Input: part model. Units: mm. Frame: model coordinates. A direction names the side the tool comes from. Give positions to 0.01 mm unless a question says otherwise; leave off trailing zeros. Loops run counter-clockwise (first coordinate to the right, second up) from the corner with the lowest first, then second, coordinate; pieces in that order, holes last. Notation, with made-up numbers: (-10, -38) -> (4, -38) arc R7 ccw to (4, -34) -> close; hole circle Ø3 at (18, -25). An arc over 180 degrees is marked (long way). Answer in a Markdown table with one row per item. Add a question column.
```python
from build123d import *

# Parameters (mm, degrees)
F0_R     = 0.3937
F1_DEPTH = 0.1778
F2_DEPTH = 1.143
F3_DEPTH = 1.524
F4_SCALE = 7.5


with BuildPart() as f1:
    # F0 (on Front) → F1 (new body, symmetric)
    with BuildSketch(Plane.XZ):
        with BuildLine():
            ThreePointArc((0, 8.2042), (-0.4130917816, 8.0330917816), (-0.5842, 7.62))
            Line((-0.5842, 7.62), (-0.5842, 0))
            ThreePointArc((-0.5842, 0), (-0.4130917816, -0.4130917816), (0, -0.5842))
            ThreePointArc((0, -0.5842), (0.4130917816, -0.4130917816), (0.5842, 0))
            Line((0.5842, 0), (0.5842, 7.62))
            ThreePointArc((0.5842, 7.62), (0.4130917816, 8.0330917816), (0, 8.2042))
        make_face()
        Circle(F0_R, mode=Mode.SUBTRACT)
        with BuildLine():
            ThreePointArc((-0.3937, 7.62), (0, 8.0137), (0.3937, 7.62))
            ThreePointArc((0.3937, 7.62), (0, 7.2263), (-0.3937, 7.62))
        make_face(mode=Mode.SUBTRACT)
    extrude(amount=F1_DEPTH, both=True)

    # F0 (on Front) → F2 (join, symmetric)
    with BuildSketch(Plane.XZ):
        Circle(F0_R)
    extrude(amount=F2_DEPTH, both=True)

    # F0 (on Front) → F3 (join)
    with BuildSketch(Plane.XZ):
        with BuildLine():
            ThreePointArc((-0.3937, 7.62), (0, 7.2263), (0.3937, 7.62))
            ThreePointArc((0.3937, 7.62), (0, 8.0137), (-0.3937, 7.62))
        make_face()
    extrude(amount=-F3_DEPTH)


with BuildPart() as f1_1:
    # F4: moved
    add(f1.part.scale(F4_SCALE))


solid = f1_1.part
```
1) Section B-B on x = -2.25. Output: boundary loops of the cut face in (y, z).
2) Section A-A on y = -0.75. Output: boundary loops of the cut face in (x, z).
3) Pull-direction query (Z, two-part tool) for faces 5 (the face through (-2.34, -5, -1.8)), 6 (the face through (0, 11.43, 57)), 7 (the face through (0, 0, 57)); classes: +Z half, -Z half, draft (parallel to the pull), parting line (faces both ways), or undercut.
4) Section C-C on y = 2. Output: boundary loops of the cut face in (x, z), and give its area (3 significant figures).
5) Section D-D on z = 29.5. Output: boundary loops of the cut face in (x, y), and give its area (3 significant figures).
6) Pin query (flat end, axial travel): pin 1 (2 mm diameter, centred on x = -1, y = 2.5, fed in from +Z); pin 2 (1 mm diameter, centred on x = -1.5, y = -1.5, fed in from +Z); pin 3 (2 mm diameter, centred on x = 3, z = 26.5, fed in from +Y). Return the tip coordinate at first contact, or that it passes through.
7) Reachability of faces 1 (the face through (-0.64, -0.657, 60.033)), 2 (the face through (-2.34, 4.9, -1.8)), 3 (the face through (0, 8.572, 0)), 4 (the face through (0, -8.572, 0)) from +Z, -Z, +X, -X, +Y, -Y: full face, straight path, thin tool, end or side. Return the list, or none.
8) Material intervals for line 1 along X through (y, z) = (-0.9, 57.15); line 2 along Y through (x, z) = (4, 33.5); line 3 along Z through (x, y) = (-1.75, 3.5), sorted ascending.
Working result:
| question | item | result |
|---|---|---|
| 1 | outline | (-8.57, -1.91) -> (-1.33, -1.91) -> (-1.33, -3.76) -> (1.33, -3.76) -> (1.33, -1.91) -> (8.57, -1.91) -> (8.57, 1.91) -> (1.33, 1.91) -> (1.33, 55.24) -> (11.43, 55.24) -> (11.43, 59.06) -> (1.33, 59.06) -> (1.33, 60.91) -> (-1.33, 60.91) -> (-1.33, 59.06) -> (0, 59.06) -> (0, 55.24) -> (-1.33, 55.24) -> (-1.33, 1.91) -> (-8.57, 1.91) -> close |
| 2 | outline | (-4.38, 0) arc R4.38 ccw to (4.38, 0) -> (4.38, 57.15) arc R4.38 ccw to (-4.38, 57.15) -> close; hole circle Ø5.91 at (0, 57.15) |
| 3 | face 5 | parting line |
| 3 | face 6 | draft |
| 3 | face 7 | undercut |
| 4 | outline | circle Ø5.91 at (0, 0); circle Ø5.91 at (0, 57.15) |
| 4 | area | 54.8 mm2 |
| 5 | outline | (-4.38, -1.33) -> (4.38, -1.33) -> (4.38, 1.33) -> (-4.38, 1.33) -> close |
| 5 | area | 23.4 mm2 |
| 6 | pin 1 | stops at z = 60.1 |
| 6 | pin 2 | stops at z = 61.41 |
| 6 | pin 3 | stops at y = 1.33 |
| 7 | face 1 | -Y |
| 7 | face 2 | +Y |
| 7 | face 3 | -Z, +X, -X, +Y |
| 7 | face 4 | +Z, -Z, +X, -X, -Y |
| 8 | line 1 | x = -4.38 to -2.95, 2.95 to 4.38 |
| 8 | line 2 | y = -1.33 to 1.33 |
| 8 | line 3 | z = -2.38 to 2.38, 54.77 to 59.53 |
